```python
from build123d import *

# Parameters (mm, degrees)
F0_W     = 490.474
F0_H     = 317.5
F0_W_2   = 465.074
F0_H_2   = 292.1
F1_DEPTH = 38.1


# Not quite as in the source:
# - the program builds the solid bodies; features that only make, move or delete a surface that nothing else refers to are left out


with BuildPart() as f1:
    # F0 (on Right) → F1 (new body, symmetric)
    with BuildSketch(Plane.YZ):
        Rectangle(F0_W, F0_H)
        Rectangle(F0_W_2, F0_H_2, mode=Mode.SUBTRACT)
    extrude(amount=F1_DEPTH, both=True)


solid = f1.part
```
Here's how the part is built. I have some questions about the finished solid (model axes, mm). A direction names the side the tool comes from. Round coordinates to 2 decimals unless told otherwise and drop trailing zeros. Write each loop counter-clockwise with the first axis right and the second up, starting at its lowest first coordinate (ties: lowest second). Pieces come first, ordered by that corner, then holes.
Q1. If we section it at C-C on z = -49.5: Write out the boundary of the cut face in (x, y), plus the area to 3 significant figures.
Q2. If we section it at A-A on y = -193: Write out the boundary of the cut face in (x, z).
Q3. Please list where these lines run through material, in increasing order: probe 1 along Y at (x, z) = (30, 36); probe 2 along Z at (x, y) = (-23.5, -21).
Q4. If we section it at B-B on x = 12.5: Write out the boundary of the cut face in (y, z), plus the area to 3 significant figures.
Q5. Which directions (+Z, -Z, +X, -X, +Y, -Y) give clear straight access to the entire face, cutting with the end or side of a thin tool? Please do faces 5 (the flat face through (1, -232.537, -2)), 6 (the flat face through (1, -3, 158.75)).
Q6. If we mould it in two halves opening along Y, with no side actions, what happens to faces 1 (the flat face through (1, 245.237, -2)), 2 (the flat face through (1, -3, 146.05)), 3 (the flat face through (1, 232.537, -2)), 4 (the flat face through (-38.1, -19, -152))? For each: +Y half, -Y half, draft (parallel to the pull), parting line (faces both ways), or undercut.
Answer below:
1. outline: (-38.1, -245.24) - (38.1, -245.24) - (38.1, -232.54) - (-38.1, -232.54) - close; (-38.1, 232.54) - (38.1, 232.54) - (38.1, 245.24) - (-38.1, 245.24) - close
1. area: 1,940 mm2
2. outline: (-38.1, -158.75) - (38.1, -158.75) - (38.1, -146.05) - (-38.1, -146.05) - close; (-38.1, 146.05) - (38.1, 146.05) - (38.1, 158.75) - (-38.1, 158.75) - close
3. probe 1: y = -245.24 to -232.54, 232.54 to 245.24
3. probe 2: z = -158.75 to -146.05, 146.05 to 158.75
4. outline: (-245.24, -158.75) - (245.24, -158.75) - (245.24, 158.75) - (-245.24, 158.75) - close; hole (-232.54, -146.05) - (232.54, -146.05) - (232.54, 146.05) - (-232.54, 146.05) - close
4. area: 19,900 mm2
5. face 5: +X, -X
5. face 6: +Z, +X, -X, +Y, -Y
6. face 1: +Y half
6. face 2: undercut
6. face 3: undercut
6. face 4: draft
